```python
from build123d import *

# Parameters (mm, degrees)
F1_DEPTH = 6.35


with BuildPart() as f1:
    # F0 (on Top) → F1 (new body)
    with BuildSketch(Plane.XY):
        with BuildLine():
            ThreePointArc((9.525, 0), (6.7351920908, 6.7351920908), (0, 9.525))
            ThreePointArc((0, 9.525), (-6.7351920908, 6.7351920908), (-9.525, 0))
            ThreePointArc((-9.525, 0), (0, -9.525), (9.525, 0))
        make_face()
        with BuildLine():
            ThreePointArc((3.175, 0), (-2.2450640303, -2.2450640303), (0, 3.175))
            ThreePointArc((0, 3.175), (2.2450640303, 2.2450640303), (3.175, 0))
        make_face(mode=Mode.SUBTRACT)
        with BuildLine():
            ThreePointArc((-9.525, 0), (-6.7351920908, 6.7351920908), (0, 9.525))
            Line((0, 9.525), (0, 13.2831632736))
            ThreePointArc((0, 13.2831632736), (-6.7351920908, 16.0729711828), (-9.525, 22.8081632736))
            Line((-9.525, 22.8081632736), (-9.525, 0))
        make_face()
        with BuildLine():
            Line((0, 13.2831632736), (0, 9.525))
            ThreePointArc((0, 9.525), (6.7351920908, 6.7351920908), (9.525, 0))
            Line((9.525, 0), (9.525, 22.8081632736))
            ThreePointArc((9.525, 22.8081632736), (6.7351920908, 16.0729711828), (0, 13.2831632736))
        make_face()
        with BuildLine():
            ThreePointArc((-9.525, 22.8081632736), (-6.7351920908, 16.0729711828), (0, 13.2831632736))
            ThreePointArc((0, 13.2831632736), (6.7351920908, 16.0729711828), (9.525, 22.8081632736))
            ThreePointArc((9.525, 22.8081632736), (0, 32.3331632736), (-9.525, 22.8081632736))
        make_face()
        with BuildLine():
            ThreePointArc((3.175, 22.8081632736), (2.2450640303, 20.5630992433), (0, 19.6331632736))
            ThreePointArc((0, 19.6331632736), (-2.2450640303, 25.0532273039), (3.175, 22.8081632736))
        make_face(mode=Mode.SUBTRACT)
    extrude(amount=F1_DEPTH)


solid = f1.part
```
Design review of the part built by this model. Coordinates are the model's own, in mm. Give positions to 0.01 mm unless a question says otherwise; leave off trailing zeros. Order: outer loops, then holes, each group sorted by start corner. A loop starts at its lowest first (then second) coordinate and runs counter-clockwise, first axis right, second up. Notation, with made-up numbers: (-6, 46) - (31, 46) arc R25 ccw to (31, 71) - close; hole circle Ø2 at (78, 39.5). An arc over 180 degrees is marked (long way). Use a Markdown table: item, result. Add a question column.
(1) Add section C-C on y = 25.5. Give the boundary of the cut face in (x, z).
(2) Wall thickness on probe 1 along Y at (x, z) = (0, 3.5) (3 decimals); probe 2 along Y at (x, z) = (-1.25, 1); probe 3 along X at (y, z) = (29.5, 1): over which ranges is each line inside the solid? List them lowest first. Write a range as [from, to].
(3) Add section D-D on x = 1. Give the boundary of the cut face in (y, z), then the cut area to 3 significant figures.
(4) Clearance check with flat-ended pins moving along their axes: P1, Ø2, axis at x = 0, y = -1.5, coming from the +Z side (1 decimal); P2, Ø1.5, axis at x = 6, z = 2.5, coming from the -Y side. State where each tip first meets the part, or that it passes through.
(5) Add section B-B on z = 4.5. Give the boundary of the cut face in (x, y) (3 decimals), then the cut area to 3 significant figures.
(6) Add section A-A on x = -1.5. Give the boundary of the cut face in (y, z).
Report:
| question | item | result |
|---|---|---|
| 1 | outline | (-9.14, 0) - (-1.68, 0) - (-1.68, 6.35) - (-9.14, 6.35) - close; (1.68, 0) - (9.14, 0) - (9.14, 6.35) - (1.68, 6.35) - close |
| 2 | probe 1 | y = [-9.525, -3.175], [3.175, 19.633], [25.983, 32.333] |
| 2 | probe 2 | y = [-9.44, -2.92], [2.92, 19.89], [25.73, 32.25] |
| 2 | probe 3 | x = [-6.78, 6.78] |
| 3 | outline | (-9.47, 0) - (-3.01, 0) - (-3.01, 6.35) - (-9.47, 6.35) - close; (3.01, 0) - (19.79, 0) - (19.79, 6.35) - (3.01, 6.35) - close; (25.82, 0) - (32.28, 0) - (32.28, 6.35) - (25.82, 6.35) - close |
| 3 | area | 189 mm² |
| 4 | P1 | passes through |
| 4 | P2 | stops at y = -7.95 |
| 5 | outline | (-9.525, 0) arc R9.525 ccw to (9.525, 0) - (9.525, 22.808) arc R9.525 ccw to (-9.525, 22.808) - close; hole circle Ø6.35 at (0, 0); hole circle Ø6.35 at (0, 22.808) |
| 5 | area | 656 mm² |
| 6 | outline | (-9.41, 0) - (-2.8, 0) - (-2.8, 6.35) - (-9.41, 6.35) - close; (2.8, 0) - (20.01, 0) - (20.01, 6.35) - (2.8, 6.35) - close; (25.61, 0) - (32.21, 0) - (32.21, 6.35) - (25.61, 6.35) - close |
